from build123d import *

# Parameters (mm, degrees)
SKETCH1_R           = 1
BOSS_EXTRUDE1_DEPTH = 8.3
FILLET1_R           = 0.15
FILLET2_R           = 0.15


with BuildPart() as part:
    # Sketch1 → Boss-Extrude1 (new body)
    with BuildSketch(Plane.XY):
        with Locations(Location((0, 0, 0), (0, 0, 180))):
            Circle(SKETCH1_R)
    extrude(amount=BOSS_EXTRUDE1_DEPTH)

    # Sketch2 → Revolve1 (revolve)
    with BuildSketch(Plane(origin=(0, 0, 0), x_dir=(1, 0, 0), z_dir=(0, 1, 0))):
        with BuildLine():
            Line((0, 0), (1.86246764, 0))
            add(Edge.make_bspline(
                [(1.86246764, 0), (1.916751975, 0.840718666), (1.329815324, 1.708509957), (0, 1.708509957)],
                knots=[0, 0, 0, 0, 1, 1, 1, 1], degree=3))
            Line((0, 1.708509957), (0, 0))
        make_face()
        with BuildLine():
            Line((0, -8.3), (1.86246764, -8.3))
            add(Edge.make_bspline(
                [(1.86246764, -8.3), (1.916751975, -9.140718666), (1.329815324, -10.008509957), (0, -10.008509957)],
                knots=[0, 0, 0, 0, 1, 1, 1, 1], degree=3))
            Line((0, -10.008509957), (0, -8.3))
        make_face()
    revolve(axis=Axis((0, 0, -4.836287687), (0, 0, 1)))

    # Fillet1
    fillet1_edges = [part.edges().sort_by_distance(p)[0] for p in [
        (-1.86246764, 0, 8.3),
    ]]
    fillet(fillet1_edges, radius=FILLET1_R)

    # Fillet2
    fillet2_edges = [part.edges().sort_by_distance(p)[0] for p in [
        (-1.86246764, 0, 0),
    ]]
    fillet(fillet2_edges, radius=FILLET2_R)


solid = part.part
Model file for the job. Use its own axes, mm. Give positions to 0.01 mm unless a question says otherwise; leave off trailing zeros. Put each result on its own line as item: value. Start each with the question number.
(1) Pull direction Z, two halves, no side cores. Call faces 1 (the face through (-1, -1, 0)), 2 (the face through (-1, -1, 8.3)): released by +Z, released by -Z, zero draft, split by the parting line, or undercut.
(2) Pin check, flat tips, straight feed: pin 1 Ø1 at (y, z) = (-1, 1) entering from -X; pin 2 Ø1.5 at (x, z) = (0.5, 4) entering from +Y; pin 3 Ø2 at (y, z) = (0, 6) entering from -X; pin 4 Ø1.7 at (x, y) = (0.5, 0.5) entering from -Z. Stop position of each tip, or through.
(3) Drill centre lines: L1, parallel to Z at x = 0.7, y = 0.9; L2, parallel to Z at x = 1.15, y = -1.2; L3, parallel to X at y = 0.85, z = 8.75. Where is each one in solid material? Low to high. Write a range as [from, to].
Results below:
1. face 1: undercut
1. face 2: undercut
2. pin 1: stops at x = -0.87
2. pin 2: stops at y = 1
2. pin 3: stops at x = -1
2. pin 4: stops at z = -1.71
3. L1: z = [-1.42, 0], [8.3, 9.72]
3. L2: z = [-0.89, 0], [8.3, 9.19]
3. L3: x = [-1.62, 1.62]
